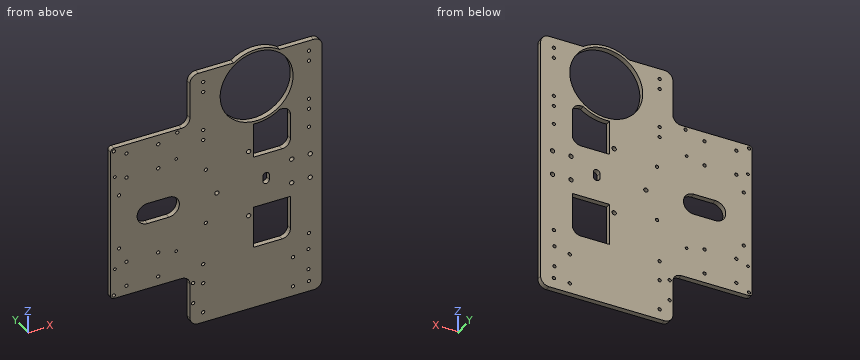
from build123d import *

# Parameters (mm, degrees)
SKETCH_1_W               = 200
SKETCH_1_H               = 250
EXTRUDE_1_DEPTH          = 5
SKETCH_2_W               = 150
SKETCH_2_H               = 100
CUT_EXTRUDE_1_DEPTH      = 10
SKETCH_3_R               = 1.55
CUT_EXTRUDE_2_DEPTH      = 10
CUT_EXTRUDE_3_DEPTH      = 10
CUT_EXTRUDE_3_DEPTH_BACK = 5
SKETCH_6_R               = 2.05
SKETCH_6_W               = 35
SKETCH_6_H               = 40
SKETCH_7_R               = 35
CUT_EXTRUDE_4_DEPTH      = 5
SKETCH_8_R               = 2.05
CUT_EXTRUDE_5_DEPTH      = 161.15617378
SKETCH_10_R              = 1.55
CUT_EXTRUDE_6_DEPTH      = 10
SKETCH_11_R              = 1.55
CUT_EXTRUDE_7_DEPTH      = 5
SKETCH_14_R              = 1.55
CUT_EXTRUDE_10_DEPTH     = 5
SKETCH_16_R              = 1.3
CUT_EXTRUDE_11_DEPTH     = 5
SKETCH_18_R              = 34.5
EXTRUDE_2_DEPTH          = 5
FILLET_1_R               = 8
SKETCH_19_R              = 1.55
CUT_EXTRUDE_12_DEPTH     = 10
SKETCH_20_R              = 1.55
CUT_EXTRUDE_13_DEPTH     = 10
CUT_EXTRUDE_14_DEPTH     = 10
FILLET_2_R               = 3
FILLET_3_R               = 8
CUT_EXTRUDE_15_DEPTH     = 10
SKETCH_23_R              = 1.55
CUT_EXTRUDE_16_DEPTH     = 10
SKETCH_24_R              = 1.55
CUT_EXTRUDE_17_DEPTH     = 10


with BuildPart() as part:
    # 草图1 → 凸台-拉伸1 (new body)
    with BuildSketch(Plane(origin=(0, 0, 0), x_dir=(1, 0, 0), z_dir=(0, 1, 0))):
        Rectangle(SKETCH_1_W, SKETCH_1_H)
    extrude(amount=EXTRUDE_1_DEPTH)

    # 草图2 → 切除-拉伸1 (cut)
    with BuildSketch(Plane(origin=(0, 5, 0), x_dir=(1, 0, 0), z_dir=(0, 1, 0))):
        with Locations((-100, 125)):
            Rectangle(SKETCH_2_W, SKETCH_2_H)
        with Locations((-100, -125)):
            Rectangle(SKETCH_2_W, SKETCH_2_H)
    extrude(amount=-CUT_EXTRUDE_1_DEPTH, mode=Mode.SUBTRACT)

    # 草图3 → 切除-拉伸2 (cut)
    with BuildSketch(Plane(origin=(0, 0, 0), x_dir=(-1, 0, 0), z_dir=(0, -1, 0))):
        with Locations(Location((85, 66, 0), (0, 0, 90))):
            Circle(SKETCH_3_R)
        with Locations(Location((55, 66, 0), (0, 0, 90))):
            Circle(SKETCH_3_R)
        with Locations(Location((55, 42, 0), (0, 0, 90))):
            Circle(SKETCH_3_R)
        with Locations(Location((85, 42, 0), (0, 0, 90))):
            Circle(SKETCH_3_R)
        with Locations(Location((55, -42, 0), (0, 0, 90))):
            Circle(SKETCH_3_R)
        with Locations(Location((85, -42, 0), (0, 0, 90))):
            Circle(SKETCH_3_R)
        with Locations(Location((55, -66, 0), (0, 0, 90))):
            Circle(SKETCH_3_R)
        with Locations(Location((85, -66, 0), (0, 0, 90))):
            Circle(SKETCH_3_R)
    extrude(amount=-CUT_EXTRUDE_2_DEPTH, mode=Mode.SUBTRACT)

    # 草图6 → 切除-拉伸3 (cut, two sides: drawn at the far end of the back side and taken through both)
    with BuildSketch(Plane(origin=(0, 0, 0), x_dir=(-1, 0, 0), z_dir=(0, -1, 0)).offset(-CUT_EXTRUDE_3_DEPTH_BACK)):
        with Locations(Location((-30.5, 32, 0), (0, 0, 270))):
            Circle(SKETCH_6_R)
        with Locations(Location((-0.5, 0, 0), (0, 0, 270))):
            Circle(SKETCH_6_R)
        with Locations(Location((-30.5, -32, 0), (0, 0, 270))):
            Circle(SKETCH_6_R)
        with Locations((-52.5, -45)):
            Rectangle(SKETCH_6_W, SKETCH_6_H)
        with Locations((-52.5, 45)):
            Rectangle(SKETCH_6_W, SKETCH_6_H)
    extrude(amount=CUT_EXTRUDE_3_DEPTH + CUT_EXTRUDE_3_DEPTH_BACK, mode=Mode.SUBTRACT)

    # 草图7 → 切除-拉伸4 (cut)
    with BuildSketch(Plane(origin=(0, 0, 0), x_dir=(-1, 0, 0), z_dir=(0, -1, 0))):
        with Locations((-38, -95)):
            Circle(SKETCH_7_R)
    extrude(amount=-CUT_EXTRUDE_4_DEPTH, mode=Mode.SUBTRACT)

    # 草图8 → 切除-拉伸5 (cut, through all)
    with BuildSketch(Plane(origin=(0, 5, 0), x_dir=(1, 0, 0), z_dir=(0, 1, 0))):
        with Locations(Location((71.25, 11.75, 0), (0, 0, 270))):
            Circle(SKETCH_8_R)
        with Locations(Location((88.75, 11.75, 0), (0, 0, 270))):
            Circle(SKETCH_8_R)
        with Locations(Location((88.75, -11.75, 0), (0, 0, 270))):
            Circle(SKETCH_8_R)
        with Locations(Location((71.25, -11.75, 0), (0, 0, 270))):
            Circle(SKETCH_8_R)
    extrude(amount=-CUT_EXTRUDE_5_DEPTH, mode=Mode.SUBTRACT)

    # 草图10 → 切除-拉伸6 (cut)
    with BuildSketch(Plane(origin=(0, 5, 0), x_dir=(1, 0, 0), z_dir=(0, 1, 0))):
        with Locations(Location((-12.5, -67, 0), (0, 0, 270))):
            Circle(SKETCH_10_R)
        with Locations(Location((-12.5, -115, 0), (0, 0, 270))):
            Circle(SKETCH_10_R)
        with Locations(Location((87.5, -67, 0), (0, 0, 270))):
            Circle(SKETCH_10_R)
        with Locations(Location((87.5, -115, 0), (0, 0, 270))):
            Circle(SKETCH_10_R)
    extrude(amount=-CUT_EXTRUDE_6_DEPTH, mode=Mode.SUBTRACT)

    # 草图11 → 切除-拉伸7 (cut)
    with BuildSketch(Plane(origin=(0, 5, 0), x_dir=(1, 0, 0), z_dir=(0, 1, 0))):
        with Locations(Location((87.5, 115, 0), (0, 0, 270))):
            Circle(SKETCH_11_R)
        with Locations(Location((87.5, 67, 0), (0, 0, 270))):
            Circle(SKETCH_11_R)
        with Locations(Location((-12.5, 115, 0), (0, 0, 270))):
            Circle(SKETCH_11_R)
        with Locations(Location((-12.5, 67, 0), (0, 0, 270))):
            Circle(SKETCH_11_R)
    extrude(amount=-CUT_EXTRUDE_7_DEPTH, mode=Mode.SUBTRACT)

    # 草图14 → 切除-拉伸10 (cut)
    with BuildSketch(Plane(origin=(0, 5, 0), x_dir=(1, 0, 0), z_dir=(0, 1, 0))):
        with Locations(Location((-92, -26.5, 0), (0, 0, 270))):
            Circle(SKETCH_14_R)
        with Locations(Location((-92, 26.5, 0), (0, 0, 270))):
            Circle(SKETCH_14_R)
        with Locations(Location((-10, 26.5, 0), (0, 0, 270))):
            Circle(SKETCH_14_R)
        with Locations(Location((-10, -26.5, 0), (0, 0, 270))):
            Circle(SKETCH_14_R)
    extrude(amount=-CUT_EXTRUDE_10_DEPTH, mode=Mode.SUBTRACT)

    # 草图16 → 切除-拉伸11 (cut)
    with BuildSketch(Plane(origin=(0, 5, 0), x_dir=(1, 0, 0), z_dir=(0, 1, 0))):
        with Locations(Location((-96, 46, 0), (0, 0, 270))):
            Circle(SKETCH_16_R)
        with Locations(Location((-38, 46, 0), (0, 0, 270))):
            Circle(SKETCH_16_R)
        with Locations(Location((-38, -46, 0), (0, 0, 270))):
            Circle(SKETCH_16_R)
        with Locations(Location((-96, -46, 0), (0, 0, 270))):
            Circle(SKETCH_16_R)
    extrude(amount=-CUT_EXTRUDE_11_DEPTH, mode=Mode.SUBTRACT)

    # 草图18 → 凸台-拉伸2 (add)
    with BuildSketch(Plane(origin=(0, 5, 0), x_dir=(1, 0, 0), z_dir=(0, 1, 0))):
        with BuildLine():
            ThreePointArc((35, -58.121822171), (12.920127592, -122.202941017), (75, -95))
            ThreePointArc((75, -95), (70.982039506, -78.231426118), (59.800807024, -65.104769392))
            ThreePointArc((59.800807024, -65.104769392), (48.0278599, -59.38480625), (35, -58.121822171))
        make_face()
        with Locations(Location((38, -95, 0), (0, 0, 270))):
            Circle(SKETCH_18_R, mode=Mode.SUBTRACT)
    extrude(amount=-EXTRUDE_2_DEPTH)

    # 圆角1
    fillet_1_edges = [part.edges().sort_by_distance(p)[0] for p in [
        (70, 2.5, -65),
        (70, 2.5, 25),
        (70, 2.5, 65),
    ]]
    fillet(fillet_1_edges, radius=FILLET_1_R)

    # 草图19 → 切除-拉伸12 (cut)
    with BuildSketch(Plane(origin=(0, 5, 0), x_dir=(1, 0, 0), z_dir=(0, 1, 0))):
        with Locations(Location((-97, 72, 0), (0, 0, 270))):
            Circle(SKETCH_19_R)
        with Locations(Location((-97, -72, 0), (0, 0, 270))):
            Circle(SKETCH_19_R)
    extrude(amount=-CUT_EXTRUDE_12_DEPTH, mode=Mode.SUBTRACT)

    # 草图20 → 切除-拉伸13 (cut)
    with BuildSketch(Plane(origin=(0, 5, 0), x_dir=(1, 0, 0), z_dir=(0, 1, 0))):
        with Locations(Location((72.498529399, 115.5, 0), (0, 0, 270))):
            Circle(SKETCH_20_R)
        with Locations(Location((72.5, 86.5, 0), (0, 0, 270))):
            Circle(SKETCH_20_R)
        with Locations(Location((87, 103, 0), (0, 0, 270))):
            Circle(SKETCH_20_R)
        with Locations(Location((87, 83, 0), (0, 0, 270))):
            Circle(SKETCH_20_R)
        with Locations(Location((-22, 103, 0), (0, 0, 270))):
            Circle(SKETCH_20_R)
        with Locations(Location((-22, 83, 0), (0, 0, 270))):
            Circle(SKETCH_20_R)
        with Locations(Location((-12.5, 86, 0), (0, 0, 270))):
            Circle(SKETCH_20_R)
    extrude(amount=-CUT_EXTRUDE_13_DEPTH, mode=Mode.SUBTRACT)

    # 草图21 → 切除-拉伸14 (cut)
    with BuildSketch(Plane(origin=(0, 5, 0), x_dir=(1, 0, 0), z_dir=(0, 1, 0))):
        with BuildLine():
            Line((-65, 10), (-45, 10))
            ThreePointArc((-45, 10), (-35, 0), (-45, -10))
            Line((-45, -10), (-65, -10))
            ThreePointArc((-65, -10), (-75, 0), (-65, 10))
        make_face()
    extrude(amount=-CUT_EXTRUDE_14_DEPTH, mode=Mode.SUBTRACT)

    # 圆角2
    fillet_2_edges = [part.edges().sort_by_distance(p)[0] for p in [
        (-100, 2.5, -75),
        (-100, 2.5, 75),
    ]]
    fillet(fillet_2_edges, radius=FILLET_2_R)

    # 圆角3
    fillet_3_edges = [part.edges().sort_by_distance(p)[0] for p in [
        (-25, 2.5, -125),
        (-25, 2.5, -75),
        (-25, 2.5, 125),
        (-25, 2.5, 75),
        (100, 2.5, 125),
        (100, 2.5, -125),
    ]]
    fillet(fillet_3_edges, radius=FILLET_3_R)

    # 草图22 → 切除-拉伸15 (cut)
    with BuildSketch(Plane(origin=(0, 0, 0), x_dir=(-1, 0, 0), z_dir=(0, -1, 0))):
        with BuildLine():
            Line((-44, 2), (-44, -3))
            ThreePointArc((-44, -3), (-47, -6), (-50, -3))
            Line((-50, -3), (-50, 2))
            ThreePointArc((-50, 2), (-47, 5), (-44, 2))
        make_face()
    extrude(amount=-CUT_EXTRUDE_15_DEPTH, mode=Mode.SUBTRACT)

    # 草图23 → 切除-拉伸16 (cut)
    with BuildSketch(Plane(origin=(0, 5, 0), x_dir=(1, 0, 0), z_dir=(0, 1, 0))):
        with Locations(Location((87.5, -39, 0), (0, 0, 270))):
            Circle(SKETCH_23_R)
        with Locations(Location((-37, -72, 0), (0, 0, 270))):
            Circle(SKETCH_23_R)
    extrude(amount=-CUT_EXTRUDE_16_DEPTH, mode=Mode.SUBTRACT)

    # 草图24 → 切除-拉伸17 (cut)
    with BuildSketch(Plane(origin=(0, 5, 0), x_dir=(1, 0, 0), z_dir=(0, 1, 0))):
        with Locations(Location((87.5, -105, 0), (0, 0, 270))):
            Circle(SKETCH_24_R)
        with Locations(Location((-12.5, -105, 0), (0, 0, 270))):
            Circle(SKETCH_24_R)
        with Locations(Location((87.5, -57, 0), (0, 0, 270))):
            Circle(SKETCH_24_R)
        with Locations(Location((-12.5, -57, 0), (0, 0, 270))):
            Circle(SKETCH_24_R)
    extrude(amount=-CUT_EXTRUDE_17_DEPTH, mode=Mode.SUBTRACT)


solid = part.part
For this review, take the finished solid that the model builds, in its own axes (mm). Give positions to 0.01 mm unless a question says otherwise; leave off trailing zeros. Loops run counter-clockwise (first coordinate to the right, second up) from the corner with the lowest first, then second, coordinate; pieces in that order, holes last.
Item 1: For line 1 along X through (y, z) = (1.25, 46); line 2 along X through (y, z) = (3.75, -12); line 3 along X through (y, z) = (3.2, -26.5), list the stretches that pass through material, from the lowest coordinate up.
Item 2: Take a section at A-A, the plane z = 95. State the section outline as (x, y) points.
Item 3: Insertion check: pin 1 (5 mm diameter, centred on x = 87, z = -83, fed in from +Y); pin 2 (3.5 mm diameter, centred on x = 88.75, z = -11.75, fed in from +Y); pin 3 (1.5 mm diameter, centred on x = 82, y = 3.5, fed in from +Z); pin 4 (1.5 mm diameter, centred on x = 45.5, y = 3, fed in from +Z). Each pin has a flat end and moves straight along its axis. Give the tip position at first contact, or say it passes through.
Item 4: Take a section at B-B, the plane x = 47. State the section outline as (y, z) points.
Item 5: Take a section at C-C, the plane y = 1.9. Give the number of separate pieces and of enclosed holes in the cut face, and give its area (3 significant figures).
Calculated:
1. line 1: x = -100 to -97.3, -94.7 to -39.3, -36.7 to 35, 70 to 100
1. line 2: x = -100 to 69.22, 73.28 to 86.72, 90.78 to 100
1. line 3: x = -100 to -93.55, -90.45 to -11.55, -8.45 to 35, 70 to 100
2. outline: (-25, 0) - (3.5, 0) - (3.5, 5) - (-25, 5) - close; (72.5, 0) - (100, 0) - (100, 5) - (72.5, 5) - close
3. pin 1: stops at y = 5
3. pin 2: passes through
3. pin 3: stops at z = 125
3. pin 4: stops at z = 131.38
4. outline: (0, -125) - (5, -125) - (5, -65) - (0, -65) - close; (0, -25) - (5, -25) - (5, -5) - (0, -5) - close; (0, 6) - (5, 6) - (5, 25) - (0, 25) - close; (0, 59.11) - (5, 59.11) - (5, 61.69) - (0, 61.69) - close; (0, 128.31) - (5, 128.31) - (5, 130.89) - (0, 130.89) - close
5. separate pieces: 1
5. enclosed holes: 51
5. area: 35,200 mm2
